Here's how the part is built. I have some questions about the finished solid (model axes, mm). Give positions to 0.01 mm unless a question says otherwise; leave off trailing zeros. Write each loop counter-clockwise with the first axis right and the second up, starting at its lowest first coordinate (ties: lowest second). Pieces come first, ordered by that corner, then holes. Notation, with made-up numbers: (81.25, 65) -> (86.25, 65) arc R18 cw to (86.25, 92) -> close; hole circle Ø2 at (-36.5, 66). An arc over 180 degrees is marked (long way). Return JSON: item names as keys, results as strings.
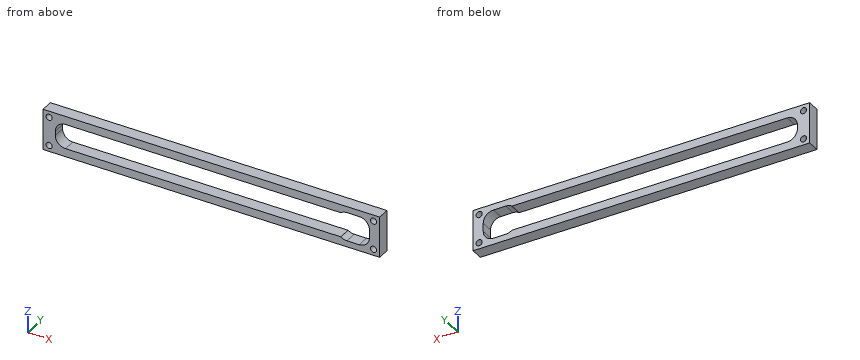
from build123d import *

# Parameters (mm, degrees)
SKETCH1_W           = 164.534777256
SKETCH1_H           = 20
SKETCH1_R           = 1.5
SKETCH1_W_2         = 152.534777256
SKETCH1_H_2         = 12
BOSS_EXTRUDE1_DEPTH = 6
CUT_EXTRUDE1_DEPTH  = 166.854432943
FILLET1_R           = 5


with BuildPart() as part:
    # Sketch1 → Boss-Extrude1 (new body)
    with BuildSketch(Plane(origin=(0, 0, 0), x_dir=(1, 0, 0), z_dir=(0, 1, 0))):
        with Locations((82.267388628, 10)):
            Rectangle(SKETCH1_W, SKETCH1_H)
        with Locations(Location((3, 17, 0), (0, 0, 270))):
            Circle(SKETCH1_R, mode=Mode.SUBTRACT)
        with Locations(Location((3, 3, 0), (0, 0, 90))):
            Circle(SKETCH1_R, mode=Mode.SUBTRACT)
        with Locations(Location((161.534777256, 3, 0), (0, 0, 270))):
            Circle(SKETCH1_R, mode=Mode.SUBTRACT)
        with Locations(Location((161.534777256, 17, 0), (0, 0, 90))):
            Circle(SKETCH1_R, mode=Mode.SUBTRACT)
        with Locations((82.267388628, 10)):
            Rectangle(SKETCH1_W_2, SKETCH1_H_2, mode=Mode.SUBTRACT)
    extrude(amount=BOSS_EXTRUDE1_DEPTH)

    # Sketch2 → Cut-Extrude1 (cut, through all)
    with BuildSketch(Plane(origin=(0, 6, 0), x_dir=(1, 0, 0), z_dir=(0, 1, 0))):
        Polygon((145.534777256, 17), (145.534777256, 16), (158.534777256, 16), (158.534777256, 4), (145.534777256, 4), (145.534777256, 3), (159.534777256, 3), (159.534777256, 17), align=None)
    extrude(amount=-CUT_EXTRUDE1_DEPTH, mode=Mode.SUBTRACT)

    # Fillet1
    # the kernel refuses this fillet: 5 mm, written as the material it adds along each edge
    with BuildSketch(Plane(origin=(159.534777256, 6, -17), x_dir=(0, 0, 1), z_dir=(0, -1, 0)), Plane(origin=(159.534777256, 6, -3), x_dir=(-1, 0, 0), z_dir=(0, -1, 0)), Plane(origin=(6, 0, -16), x_dir=(0, 0, 1), z_dir=(0, 1, 0))) as fillet1_piece_1:
        with BuildLine():
            CenterArc((FILLET1_R, FILLET1_R), FILLET1_R, 180, 90)
            Line((0, FILLET1_R), (-FILLET1_R * 0.02, FILLET1_R))
            Line((-FILLET1_R * 0.02, FILLET1_R), (-FILLET1_R * 0.02, -FILLET1_R * 0.02))
            Line((-FILLET1_R * 0.02, -FILLET1_R * 0.02), (FILLET1_R, -FILLET1_R * 0.02))
            Line((FILLET1_R, -FILLET1_R * 0.02), (FILLET1_R, 0))
        make_face()
    extrude(amount=6)
    with BuildSketch(Plane(origin=(145.534777256, 6, -17), x_dir=(1, 0, 0), z_dir=(0, -1, 0))) as fillet1_piece_2:
        with BuildLine():
            CenterArc((3, 5), FILLET1_R, 233.130102354, 36.869897646)
            Line((0, 1), (-0.06, 0.92))
            ThreePointArc((-0.06, 0.92), (-0.1, 0.5), (-0.1, 0))
            Line((-0.1, 0), (0, -0.1))
            Line((0, -0.1), (3, -0.1))
            Line((3, -0.1), (3, 0))
        make_face()
    extrude(amount=6)
    with BuildSketch(Plane(origin=(145.534777256, 6, -3), x_dir=(0, 0, -1), z_dir=(0, -1, 0))) as fillet1_piece_3:
        with BuildLine():
            CenterArc((5, 3), FILLET1_R, 180, 36.869897646)
            Line((0, 3), (-0.1, 3))
            Line((-0.1, 3), (-0.1, 0))
            Line((-0.1, 0), (0, -0.1))
            ThreePointArc((0, -0.1), (0.5, -0.1), (0.92, -0.06))
            Line((0.92, -0.06), (1, 0))
        make_face()
    extrude(amount=6)
    with BuildSketch(Plane(origin=(6, 0, -4), x_dir=(0, 0, -1), z_dir=(0, 1, 0))) as fillet1_piece_4:
        with BuildLine():
            CenterArc((FILLET1_R, -FILLET1_R), FILLET1_R, 90, 90)
            Line((0, -FILLET1_R), (-FILLET1_R * 0.02, -FILLET1_R))
            Line((-FILLET1_R * 0.02, -FILLET1_R), (-FILLET1_R * 0.02, FILLET1_R * 0.02))
            Line((-FILLET1_R * 0.02, FILLET1_R * 0.02), (FILLET1_R, FILLET1_R * 0.02))
            Line((FILLET1_R, FILLET1_R * 0.02), (FILLET1_R, 0))
        make_face()
    extrude(amount=6)


solid = part.part
1. Suppose I cut it at D-D, the plane y = 2.5. List the corners of the cut face in (x, z) for me, and give its area (3 significant figures).
Taken from the geometry:
{"outline": "(0, -20) -> (164.53, -20) -> (164.53, 0) -> (0, 0) -> close; hole circle Ø3 at (3, -17); hole circle Ø3 at (3, -3); hole (6, -11) arc R5 ccw to (11, -16) -> (145.53, -16) arc R5 ccw to (148.53, -17) -> (154.53, -17) arc R5 ccw to (159.53, -12) -> (159.53, -8) arc R5 ccw to (154.53, -3) -> (148.53, -3) arc R5 ccw to (145.53, -4) -> (11, -4) arc R5 ccw to (6, -9) -> close; hole circle Ø3 at (161.53, -17); hole circle Ø3 at (161.53, -3)", "area": "1,420 mm²"}
2. If I drill on line 1 (Z direction, x = 42, y = 4.3); line 2 (X direction, y = 1.8, z = -9); line 3 (Z direction, x = 154, y = 4.9), over which ranges is the centre line in solid material (lowest first)? Write a range as [from, to].
Taken from the geometry:
{"line 1": "z = [-20, -16], [-4, 0]", "line 2": "x = [0, 6], [159.53, 164.53]", "line 3": "z = [-20, -17], [-3, 0]"}
3. Suppose I cut it at C-C, the plane z = -6.5. List the corners of the cut face in (x, y) for me, and give its area (3 significant figures).
Taken from the geometry:
{"outline": "(0, 0) -> (6.67, 0) -> (6.67, 6) -> (0, 6) -> close; (159.3, 0) -> (164.53, 0) -> (164.53, 6) -> (159.3, 6) -> close", "area": "71.4 mm²"}
4. For pin 1 Ø1 at (x, y) = (51, 3) entering from +Z, with a flat end and sliding along its axis, tell me the tip position at first contact or that it passes through.
Taken from the geometry:
{"pin 1": "stops at z = 0"}
5. Suppose I cut it at B-B, the plane x = 3. List the corners of the cut face in (y, z) for me, and give its area (3 significant figures).
Taken from the geometry:
{"outline": "(0, -20) -> (6, -20) -> (6, -18.5) -> (0, -18.5) -> close; (0, -15.5) -> (6, -15.5) -> (6, -4.5) -> (0, -4.5) -> close; (0, -1.5) -> (6, -1.5) -> (6, 0) -> (0, 0) -> close", "area": "84.0 mm²"}
6. Suppose I cut it at A-A, the plane x = 20. List the corners of the cut face in (y, z) for me.
Taken from the geometry:
{"outline": "(0, -20) -> (6, -20) -> (6, -16) -> (0, -16) -> close; (0, -4) -> (6, -4) -> (6, 0) -> (0, 0) -> close"}
